```python
from build123d import *

# Parameters (mm, degrees)
EXTRUDE_1_DEPTH     = 16.5
SKETCH_3_W          = 10
SKETCH_3_H          = 16.5
CUT_EXTRUDE_2_DEPTH = 3
SKETCH_4_W          = 11.896315449
SKETCH_4_H          = 29.084641161
CUT_EXTRUDE_3_DEPTH = 48.945933091
SKETCH_5_R          = 2
CUT_EXTRUDE_4_DEPTH = 48.945933091
SKETCH_6_W          = 10
SKETCH_6_H          = 23
EXTRUDE_2_DEPTH     = 3
SKETCH_7_R          = 2.5
CUT_EXTRUDE_5_DEPTH = 3
EXTRUDE_START       = 3
SKETCH_8_R          = 2
SKETCH_8_W          = 6
SKETCH_8_H          = 26
EXTRUDE_3_DEPTH     = 3
SKETCH_9_R          = 2.5
CUT_EXTRUDE_6_DEPTH = 3
SKETCH_10_W         = 74.694005649
SKETCH_10_H         = 52.095093629
CUT_EXTRUDE_7_DEPTH = 116.604119736
SKETCH_13_R         = 2
EXTRUDE_4_DEPTH     = 19.5
SKETCH_14_W         = 6
SKETCH_14_H         = 41.5
CUT_EXTRUDE_9_DEPTH = 3
SKETCH_15_W         = 23
SKETCH_15_H         = 10
SKETCH_15_R         = 2.5
EXTRUDE_5_DEPTH     = 3
SKETCH_16_W         = 3
SKETCH_16_H         = 10
EXTRUDE_6_DEPTH     = 16.5


with BuildPart() as part:
    # 草图1 → 凸台-拉伸1 (new body)
    with BuildSketch(Plane.XY):
        Polygon((0, 0), (26.75, 0), (26.75, -20), (36.75, -20), (36.75, -26), (20.75, -26), (20.75, -6), (0, -6), (-20.75, -6), (-20.75, -26), (-36.75, -26), (-36.75, -20), (-26.75, -20), (-26.75, 0), align=None)
    extrude(amount=EXTRUDE_1_DEPTH)

    # 草图3 → 切除-拉伸2 (cut)
    with BuildSketch(Plane(origin=(0, -20, 0), x_dir=(1, 0, 0), z_dir=(0, 1, 0))):
        with Locations((31.75, -8.25)):
            Rectangle(SKETCH_3_W, SKETCH_3_H)
    extrude(amount=-CUT_EXTRUDE_2_DEPTH, mode=Mode.SUBTRACT)

    # 草图4 → 切除-拉伸3 (cut, through all)
    with BuildSketch(Plane.XY.offset(16.5)):
        with Locations((-32.698157724, -14.542320581)):
            Rectangle(SKETCH_4_W, SKETCH_4_H)
    extrude(amount=-CUT_EXTRUDE_3_DEPTH, mode=Mode.SUBTRACT)

    # 草图5 → 切除-拉伸4 (cut, through all)
    with BuildSketch(Plane(origin=(0, 0, 0), x_dir=(-1, 0, 0), z_dir=(0, 0, -1))):
        with Locations((-24.3, -11)):
            Circle(SKETCH_5_R)
        with Locations((-24.3, -21)):
            Circle(SKETCH_5_R)
        with Locations(Location((24.3, -21, 0), (0, 0, 180))):
            Circle(SKETCH_5_R)
        with Locations(Location((24.3, -11, 0), (0, 0, 180))):
            Circle(SKETCH_5_R)
    extrude(amount=-CUT_EXTRUDE_4_DEPTH, mode=Mode.SUBTRACT)

    # 草图6 → 凸台-拉伸2 (add)
    with BuildSketch(Plane(origin=(0, 0, 0), x_dir=(-1, 0, 0), z_dir=(0, 0, -1))):
        with Locations((-31.75, -34.5)):
            Rectangle(SKETCH_6_W, SKETCH_6_H)
    extrude(amount=EXTRUDE_2_DEPTH)

    # 草图7 → 切除-拉伸5 (cut)
    with BuildSketch(Plane(origin=(0, 0, -3), x_dir=(-1, 0, 0), z_dir=(0, 0, -1))):
        with Locations((-31.75, -36)):
            Circle(SKETCH_7_R)
    extrude(amount=-CUT_EXTRUDE_5_DEPTH, mode=Mode.SUBTRACT)

    # 草图8 → 凸台-拉伸3 (add)
    # profile 1 of 2: a face of its own
    with BuildSketch(Plane(origin=(0, 0, 0), x_dir=(-1, 0, 0), z_dir=(0, 0, -1)).offset(EXTRUDE_START)):
        Polygon((26.75, 0), (20.75, 0), (20.75, -46), (26.75, -46), (30.75, -46), (30.75, -26), (26.75, -26), align=None)
        with Locations((24.3, -21)):
            Circle(SKETCH_8_R, mode=Mode.SUBTRACT)
        with Locations((24.3, -11)):
            Circle(SKETCH_8_R, mode=Mode.SUBTRACT)
    # profile 2 of 2: a face of its own
    with BuildSketch(Plane(origin=(0, 0, 0), x_dir=(-1, 0, 0), z_dir=(0, 0, -1)).offset(EXTRUDE_START)):
        with Locations((-23.75, -13)):
            Rectangle(SKETCH_8_W, SKETCH_8_H)
        with Locations((-24.3, -11)):
            Circle(SKETCH_8_R, mode=Mode.SUBTRACT)
        with Locations((-24.3, -21)):
            Circle(SKETCH_8_R, mode=Mode.SUBTRACT)
    extrude(amount=-EXTRUDE_3_DEPTH)

    # 草图9 → 切除-拉伸6 (cut)
    with BuildSketch(Plane(origin=(0, 0, -3), x_dir=(-1, 0, 0), z_dir=(0, 0, -1))):
        with Locations((25.75, -36)):
            Circle(SKETCH_9_R)
    extrude(amount=-CUT_EXTRUDE_6_DEPTH, mode=Mode.SUBTRACT)

    # 镜向1: part across plane


with BuildPart() as part_1:
    add(part.part)
    add(part.part.mirror(Plane(origin=(36.75, -20, 16.5), x_dir=(0, 0, 1), z_dir=(-1, 0, 0))))

    # 草图10 → 切除-拉伸7 (cut, through all)
    with BuildSketch(Plane(origin=(0, 0, -3), x_dir=(-1, 0, 0), z_dir=(0, 0, -1))):
        with Locations((0.597002825, -19.952453186)):
            Rectangle(SKETCH_10_W, SKETCH_10_H)
    extrude(amount=-CUT_EXTRUDE_7_DEPTH, mode=Mode.SUBTRACT)

    # 草图13 → 凸台-拉伸4 (add)
    with BuildSketch(Plane(origin=(0, 0, -3), x_dir=(-1, 0, 0), z_dir=(0, 0, -1))):
        Polygon((-24.75, -6), (-50.75, -6), (-50.75, 47.5), (-24.75, 47.5), (-24.75, 41.5), (-44.75, 41.5), (-44.75, 0), (-24.75, 0), align=None)
        with Locations((-29.75, -3.55)):
            Circle(SKETCH_13_R, mode=Mode.SUBTRACT)
        with Locations((-39.75, -3.55)):
            Circle(SKETCH_13_R, mode=Mode.SUBTRACT)
        with Locations(Location((-39.75, 45.05, 0), (0, 0, 180))):
            Circle(SKETCH_13_R, mode=Mode.SUBTRACT)
        with Locations(Location((-29.75, 45.05, 0), (0, 0, 180))):
            Circle(SKETCH_13_R, mode=Mode.SUBTRACT)
    extrude(amount=-EXTRUDE_4_DEPTH)

    # 草图14 → 切除-拉伸9 (cut)
    with BuildSketch(Plane(origin=(0, 0, -3), x_dir=(-1, 0, 0), z_dir=(0, 0, -1))):
        with Locations((-47.75, 20.75)):
            Rectangle(SKETCH_14_W, SKETCH_14_H)
    extrude(amount=-CUT_EXTRUDE_9_DEPTH, mode=Mode.SUBTRACT)

    # 草图15 → 凸台-拉伸5 (add)
    with BuildSketch(Plane(origin=(0, 0, -3), x_dir=(-1, 0, 0), z_dir=(0, 0, -1))):
        with Locations((-16.25, -11)):
            Rectangle(SKETCH_15_W, SKETCH_15_H)
        with Locations((-14.75, -11)):
            Circle(SKETCH_15_R, mode=Mode.SUBTRACT)
    extrude(amount=-EXTRUDE_5_DEPTH)

    # 草图16 → 凸台-拉伸6 (add)
    with BuildSketch(Plane.XY):
        with Locations((26.25, -11)):
            Rectangle(SKETCH_16_W, SKETCH_16_H)
    extrude(amount=EXTRUDE_6_DEPTH)


solid = part_1.part
```
Geometry check sheet. Reference: the model listing, model coordinates, mm. A direction names the side the tool comes from. Coordinates: 2 decimals unless noted, no trailing zeros. Loops run counter-clockwise (first coordinate to the right, second up) from the corner with the lowest first, then second, coordinate; pieces in that order, holes last.
Item 1: Access from +Z, -Z, +X, -X, +Y, -Y to the whole of each face (thin tool, end or side, straight path). Record for faces 4 (the face through (17, -13, 0)), 5 (the face through (48, 21, 0)), 6 (the face through (74, -6, 8)), 7 (the face through (37, -6, 7)), 8 (the face through (102, -26, -2)).
Item 2: Sectioned sample at C-C, the plane z = 3.5. Count the separate pieces of the cut face and the enclosed holes in it, then the cut area to 3 significant figures.
Item 3: Thickness scan on line 1 (Y direction, x = 49.2, z = 9.75); line 2 (Y direction, x = 97.8, z = 4.5); line 3 (Y direction, x = 29.75, z = 10.75). Record the ranges inside material, lowest first.
Item 4: Release check for a two-part mould opening along Y. For faces 1 (the face through (41.748, -3.462, 6.614)), 2 (the face through (99, -46, -2)), 3 (the face through (38, 47.5, 7)) record: released by +Y, released by -Y, zero draft, split by the parting line, or undercut.
Item 5: Sectioned sample at A-A, the plane y = -36. Record the boundary of the cut face in (x, z).
Item 6: Go/stop test with flat-tipped pins: pin 1 Ø5 at (x, y) = (10.5, -13) entering from +Z; pin 2 Ø0.9 at (x, z) = (17, -1.5) entering from +Y; pin 3 Ø2.5 at (x, y) = (97.8, -11) entering from +Z; pin 4 Ø5 at (x, z) = (94, 7) entering from +Y. Record where each tip stops, or that it passes through.
Item 7: Sectioned sample at D-D, the plane y = -3.55. Record the boundary of the cut face in (x, z).
Item 8: Sectioned sample at B-B, the plane x = 43. Record the boundary of the cut face in (y, z).
Check result:
1. face 4: +Z, -X, +Y, -Y
1. face 5: -Z, +X, -X
1. face 6: +Z, -Z, -Y
1. face 7: +Z, -Z
1. face 8: +Z, -Z, +X, +Y
2. separate pieces: 1
2. enclosed holes: 8
2. area: 1,060 mm2
3. line 1: y = -26 to -23, -19 to -13, -9 to 47.5
3. line 2: y = -26 to -23, -19 to -13, -9 to 0
3. line 3: y = -6 to -5.55, -1.55 to 0, 41.5 to 43.05, 47.05 to 47.5
4. face 1: undercut
4. face 2: released by -Y
4. face 3: released by +Y
5. outline: (36.75, -3) - (39.25, -3) - (39.25, 0) - (36.75, 0) - close; (44.25, -3) - (46.75, -3) - (46.75, 0) - (44.25, 0) - close; (94.25, -3) - (96.75, -3) - (96.75, 0) - (94.25, 0) - close; (101.75, -3) - (104.25, -3) - (104.25, 0) - (101.75, 0) - close
6. pin 1: stops at z = 0
6. pin 2: stops at y = -6
6. pin 3: passes through
6. pin 4: stops at y = 0
7. outline: (24.75, -3) - (27.75, -3) - (27.75, 16.5) - (24.75, 16.5) - close; (31.75, -3) - (37.75, -3) - (37.75, 16.5) - (31.75, 16.5) - close; (41.75, -3) - (52.75, -3) - (52.75, 0) - (94.25, 0) - (94.25, -3) - (100.25, -3) - (100.25, 16.5) - (41.75, 16.5) - close
8. outline: (-46, -3) - (-38.17, -3) - (-38.17, 0) - (-46, 0) - close; (-33.83, -3) - (-23, -3) - (-23, 16.5) - (-26, 16.5) - (-26, 0) - (-33.83, 0) - close; (-6, -3) - (0, -3) - (0, 16.5) - (-6, 16.5) - close; (41.5, -3) - (47.5, -3) - (47.5, 16.5) - (41.5, 16.5) - close
